Can you work these out from the model? Positions are in its coordinate system, mm. Face numbers are marked on the shaded views. Give positions to 0.01 mm unless a question says otherwise; leave off trailing zeros. Loops run counter-clockwise (first coordinate to the right, second up) from the corner with the lowest first, then second, coordinate; pieces in that order, holes last. Notation, with made-up numbers: M -13,71.5 L 20,71.5 A22 ccw 20,96.5 Z; hole C -28,4.5 d3. An arc over 180 degrees is marked long. Put each result on its own line as item: value. Start each with the question number.
1) Imagine slicing it at A-A (z = -20). Write out the boundary of the cut face in (x, y).
2) Imagine slicing it at B-B (x = 20). Write out the boundary of the cut face in (y, z), then the cut area to 3 significant figures.
3) Please list where these lines run through material, in increasing order: line 1 along Z through (x, y) = (4, 5.25); line 2 along Z through (x, y) = (4, 3.5); line 3 along X through (y, z) = (3, -4). Write a range as from..to.
4) If we mould it in two halves opening along X, with no side actions, what happens to the marked faces 1, 2, 3 and 4? For each: +X half, -X half, draft (parallel to the pull), parting line (faces both ways), or undercut.
5) Imagine slicing it at C-C (x = 4). Write out the boundary of the cut face in (y, z).
6) Imagine slicing it at D-D (z = -36). Write out the boundary of the cut face in (x, y).
7) For P1, Ø2.5, axis at x = 36, z = -4, coming from the -Y side; P2, Ø12, axis at x = 24, z = -30, coming from the +Y side, each with a flat end and sliding along its axis, tell me the tip position at first contact or that it passes through.
from build123d import *

# Parameters (mm, degrees)
SKETCH1_W           = 40
SKETCH1_H           = 40
BOSS_EXTRUDE1_DEPTH = 8.5
SKETCH2_R           = 1.3525
SKETCH2_R_2         = 2.1
CUT_EXTRUDE1_DEPTH  = 9.5
SKETCH3_R           = 3.5
CUT_EXTRUDE2_DEPTH  = 4.25
CUT_EXTRUDE3_DEPTH  = 4.25
FILLET1_R           = 1


with BuildPart() as part:
    # Sketch1 → Boss-Extrude1 (new body)
    with BuildSketch(Plane(origin=(0, 0, 0), x_dir=(1, 0, 0), z_dir=(0, 1, 0))):
        with Locations((20, 20)):
            Rectangle(SKETCH1_W, SKETCH1_H)
    extrude(amount=BOSS_EXTRUDE1_DEPTH)

    # Sketch2 → Cut-Extrude1 (cut, through all)
    with BuildSketch(Plane(origin=(0, 8.5, 0), x_dir=(1, 0, 0), z_dir=(0, 1, 0))):
        with Locations((4, 4)):
            Circle(SKETCH2_R)
        with Locations((36, 4)):
            Circle(SKETCH2_R)
        with Locations((36, 36)):
            Circle(SKETCH2_R)
        with Locations((4, 36)):
            Circle(SKETCH2_R)
        with Locations((20, 20)):
            Circle(SKETCH2_R_2)
    extrude(amount=-CUT_EXTRUDE1_DEPTH, mode=Mode.SUBTRACT)

    # Sketch3 → Cut-Extrude2 (cut)
    with BuildSketch(Plane(origin=(0, 8.5, 0), x_dir=(1, 0, 0), z_dir=(0, 1, 0))):
        with Locations((20, 20)):
            Circle(SKETCH3_R)
    extrude(amount=-CUT_EXTRUDE2_DEPTH, mode=Mode.SUBTRACT)

    # Sketch4 → Cut-Extrude3 (cut)
    with BuildSketch(Plane(origin=(0, 8.5, 0), x_dir=(1, 0, 0), z_dir=(0, 1, 0))):
        Polygon((0, 8), (8, 8), (8, 0), (32, 0), (32, 8), (40, 8), (40, 32), (32, 32), (32, 40), (8, 40), (8, 32), (0, 32), align=None)
    extrude(amount=-CUT_EXTRUDE3_DEPTH, mode=Mode.SUBTRACT)

    # Fillet1
    fillet1_edges = [part.edges().sort_by_distance(p)[0] for p in [
        (0, 4.25, -40),
        (40, 4.25, -40),
        (40, 4.25, 0),
        (0, 4.25, 0),
        (0, 6.375, -8),
        (0, 6.375, -32),
        (8, 6.375, -32),
        (8, 6.375, -40),
        (32, 6.375, -40),
        (32, 6.375, -32),
        (40, 6.375, -32),
        (40, 6.375, -8),
        (32, 6.375, -8),
        (32, 6.375, 0),
        (8, 6.375, 0),
        (8, 6.375, -8),
    ]]
    fillet(fillet1_edges, radius=FILLET1_R)


solid = part.part
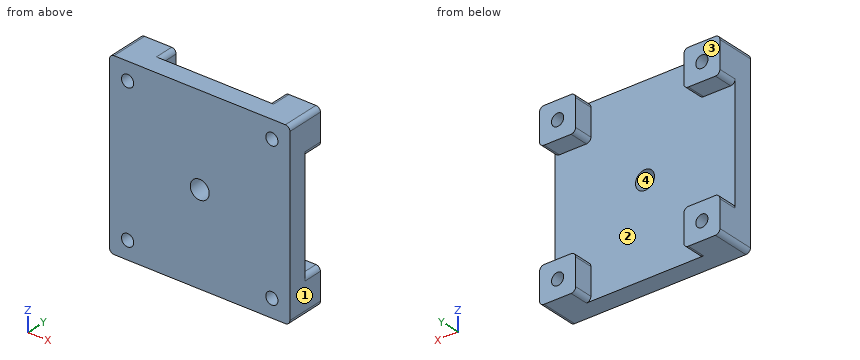
Recorded:
1. outline: M 0,0 L 17.9,0 L 17.9,4.25 L 0,4.25 Z; M 22.1,0 L 40,0 L 40,4.25 L 22.1,4.25 Z
2. outline: M 0,-40 L 4.25,-40 L 4.25,-22.1 L 0,-22.1 Z; M 0,-17.9 L 4.25,-17.9 L 4.25,0 L 0,0 Z
2. area: 152 mm²
3. line 1: -40..-37.35, -34.65..-32, -8..-5.35, -2.65..0
3. line 2: -40..-37.35, -34.65..-5.35, -2.65..0
3. line 3: 0..2.65, 5.35..34.65, 37.35..40
4. face 1: +X half
4. face 2: undercut
4. face 3: draft
4. face 4: undercut
5. outline: M 0,-40 L 8.5,-40 L 8.5,-37.35 L 0,-37.35 Z; M 0,-34.65 L 8.5,-34.65 L 8.5,-32 L 4.25,-32 L 4.25,-8 L 8.5,-8 L 8.5,-5.35 L 0,-5.35 Z; M 0,-2.65 L 8.5,-2.65 L 8.5,0 L 0,0 Z
6. outline: M 0,0 L 2.65,0 L 2.65,8.5 L 0,8.5 Z; M 5.35,0 L 34.65,0 L 34.65,8.5 L 32,8.5 L 32,4.25 L 8,4.25 L 8,8.5 L 5.35,8.5 Z; M 37.35,0 L 40,0 L 40,8.5 L 37.35,8.5 Z
7. P1: through
7. P2: y = 4.25
